from build123d import *

# Parameters (mm, degrees)
BOSS_EXTRU_1_DEPTH      = 35
COQUE1_T                = -2
ESQUISSE2_W             = 12
ESQUISSE2_H             = 12
ENL_V_MAT_EXTRU_1_DEPTH = 10
ESQUISSE3_W             = 30
ESQUISSE3_H             = 9
ENL_V_MAT_EXTRU_2_DEPTH = 10
ESQUISSE4_W             = 50
ESQUISSE4_H             = 12
ENL_V_MAT_EXTRU_3_DEPTH = 10
CONG_1_R                = 3
CONG_2_R                = 1
CONG_3_R                = 2
ESQUISSE5_R             = 3
ESQUISSE5_R_2           = 1.6
BOSS_EXTRU_2_DEPTH      = 10
CONG_4_R                = 2


with BuildPart() as part:
    # Esquisse1 → Boss.-Extru.1 (new body)
    with BuildSketch(Plane.XY):
        with BuildLine():
            Line((5, 0), (190, 0))
            ThreePointArc((190, 0), (193.535533906, 1.464466094), (195, 5))
            Line((195, 5), (195, 115))
            ThreePointArc((195, 115), (193.535533906, 118.535533906), (190, 120))
            Line((190, 120), (5, 120))
            ThreePointArc((5, 120), (1.464466094, 118.535533906), (0, 115))
            Line((0, 115), (0, 5))
            ThreePointArc((0, 5), (1.464466094, 1.464466094), (5, 0))
        make_face()
    extrude(amount=BOSS_EXTRU_1_DEPTH)

    # Coque1
    coque1_openings = [part.faces().sort_by_distance(p)[0] for p in [
        (97.5, 60, 35),
    ]]
    offset(amount=COQUE1_T, openings=coque1_openings, kind=Kind.INTERSECTION)

    # Esquisse2 → Enlèv. mat.-Extru.1 (cut)
    with BuildSketch(Plane(origin=(0, 120, 0), x_dir=(1, 0, 0), z_dir=(0, 1, 0))):
        with Locations((155.5, -19)):
            Rectangle(ESQUISSE2_W, ESQUISSE2_H)
        with BuildLine():
            Line((52, -10), (138, -10))
            ThreePointArc((138, -10), (139.414213562, -10.585786438), (140, -12))
            Line((140, -12), (140, -23))
            ThreePointArc((140, -23), (139.414213562, -24.414213562), (138, -25))
            Line((138, -25), (52, -25))
            ThreePointArc((52, -25), (50.585786438, -24.414213562), (50, -23))
            Line((50, -23), (50, -12))
            ThreePointArc((50, -12), (50.585786438, -10.585786438), (52, -10))
        make_face()
    extrude(amount=-ENL_V_MAT_EXTRU_1_DEPTH, mode=Mode.SUBTRACT)

    # Esquisse3 → Enlèv. mat.-Extru.2 (cut)
    with BuildSketch(Plane(origin=(0, 120, 0), x_dir=(1, 0, 0), z_dir=(0, 1, 0))):
        with Locations((71, -29.5)):
            Rectangle(ESQUISSE3_W, ESQUISSE3_H)
    extrude(amount=-ENL_V_MAT_EXTRU_2_DEPTH, mode=Mode.SUBTRACT)

    # Esquisse4 → Enlèv. mat.-Extru.3 (cut)
    with BuildSketch(Plane.XZ):
        with Locations((45, 18)):
            Rectangle(ESQUISSE4_W, ESQUISSE4_H)
    extrude(amount=-ENL_V_MAT_EXTRU_3_DEPTH, mode=Mode.SUBTRACT)

    # Congé1
    cong_1_edges = [part.edges().sort_by_distance(p)[0] for p in [
        (86, 119, 25),
        (56, 119, 25),
        (56, 119, 34),
        (86, 119, 34),
    ]]
    fillet(cong_1_edges, radius=CONG_1_R)

    # Congé2
    cong_2_edges = [part.edges().sort_by_distance(p)[0] for p in [
        (149.5, 119, 25),
        (149.5, 119, 13),
        (161.5, 119, 13),
        (161.5, 119, 25),
    ]]
    fillet(cong_2_edges, radius=CONG_2_R)

    # Congé3
    cong_3_edges = [part.edges().sort_by_distance(p)[0] for p in [
        (20, 1, 12),
        (20, 1, 24),
        (70, 1, 24),
        (70, 1, 12),
    ]]
    fillet(cong_3_edges, radius=CONG_3_R)

    # Esquisse5 → Boss.-Extru.2 (add)
    # profile 1 of 4: a face of its own
    with BuildSketch(Plane.XY.offset(2)):
        with Locations((10.5, 113)):
            Circle(ESQUISSE5_R)
        with Locations((10.5, 113)):
            Circle(ESQUISSE5_R_2, mode=Mode.SUBTRACT)
    # profile 2 of 4: a face of its own
    with BuildSketch(Plane.XY.offset(2)):
        with Locations((73.5, 14)):
            Circle(ESQUISSE5_R)
        with Locations((73.5, 14)):
            Circle(ESQUISSE5_R_2, mode=Mode.SUBTRACT)
    # profile 3 of 4: a face of its own
    with BuildSketch(Plane.XY.offset(2)):
        with Locations((144.5, 34)):
            Circle(ESQUISSE5_R)
        with Locations((144.5, 34)):
            Circle(ESQUISSE5_R_2, mode=Mode.SUBTRACT)
    # profile 4 of 4: a face of its own
    with BuildSketch(Plane.XY.offset(2)):
        with Locations((183.5, 112)):
            Circle(ESQUISSE5_R)
        with Locations((183.5, 112)):
            Circle(ESQUISSE5_R_2, mode=Mode.SUBTRACT)
    extrude(amount=BOSS_EXTRU_2_DEPTH)

    # Congé4
    cong_4_edges = [part.edges().sort_by_distance(p)[0] for p in [
        (7.5, 113, 2),
        (70.5, 14, 2),
        (141.5, 34, 2),
        (180.5, 112, 2),
    ]]
    fillet(cong_4_edges, radius=CONG_4_R - 0.0001)  # a hair under: the kernel refuses the full size


solid = part.part
Geometry: final body of the model. Coordinates: model frame, mm. A direction names the side the tool comes from. Give positions to 0.01 mm unless a question says otherwise; leave off trailing zeros. Order: outer loops, then holes, each group sorted by start corner. A loop starts at its lowest first (then second) coordinate and runs counter-clockwise, first axis right, second up. Notation, with made-up numbers: (-0.75, -2) -> (32.25, -2) arc R20 cw to (32.25, 7) -> close; hole circle Ø6 at (-29, 74.25). An arc over 180 degrees is marked (long way). Answer as a JSON object with one key per item and string values.
Q1. Draft query along Y for faces 1 (the flat face through (96, 61, 2)), 2 (the cylindrical face through (2, 119, 17)), 3 (the flat face through (75, 13, 12)), 4 (the flat face through (12, 112, 12)). Return one class per face: released by +Y, released by -Y, zero draft, split by the parting line, or undercut.
Entries:
{"face 1": "undercut", "face 2": "released by +Y", "face 3": "zero draft", "face 4": "undercut"}
Q2. Section B-B (x = 33). Output: boundary loops of the cut face in (y, z).
Entries:
{"outline": "(0, 0) -> (120, 0) -> (120, 35) -> (118, 35) -> (118, 2) -> (2, 2) -> (2, 12) -> (0, 12) -> close; (0, 24) -> (2, 24) -> (2, 35) -> (0, 35) -> close"}
Q3. Section A-A (z = 7). State how many separate pieces and enclosed holes the cut face has, plus the area to 3 significant figures.
Entries:
{"separate pieces": "5", "enclosed holes": "5", "area": "1,310 mm^2"}
Q4. Material intervals for probe 1 along Y at (x, z) = (144.5, 5.25); probe 2 along Y at (x, z) = (73.5, 10.25); probe 3 along Y at (x, z) = (10.5, 5.5), sorted ascending.
Entries:
{"probe 1": "y = 0 to 2, 31 to 32.4, 35.6 to 37, 118 to 120", "probe 2": "y = 0 to 2, 11 to 12.4, 15.6 to 17", "probe 3": "y = 0 to 2, 110 to 111.4, 114.6 to 116, 118 to 120"}
Q5. Section C-C (y = 78). Output: boundary loops of the cut face in (x, z).
Entries:
{"outline": "(0, 0) -> (195, 0) -> (195, 35) -> (193, 35) -> (193, 2) -> (2, 2) -> (2, 35) -> (0, 35) -> close"}
Q6. Access query for faces 5 (the flat face through (2, 61, 18)), 6 (the cylindrical face through (193, 1, 17)). Directions: +Z, -Z, +X, -X, +Y, -Y. A direction counts if a zero-diameter tool reaches every point of the face in a straight line with its end or side. Return the directions, or none.
Entries:
{"face 5": "+Z", "face 6": "+Z, -Z, +X, -Y"}
Q7. First-contact query: pin 1 (3 mm diameter, centred on x = 63.5, z = 29.5, fed in from +Y); pin 2 (6.5 mm diameter, centred on x = 184, y = 111, fed in from +Z); pin 3 (1 mm diameter, centred on y = 119, z = 19, fed in from -X). Flat tips, straight axial feed; report the tip coordinate or a pass-through.
Entries:
{"pin 1": "stops at y = 2", "pin 2": "stops at z = 12", "pin 3": "stops at x = 1.43"}
